Input: part model. Units: mm. Frame: model coordinates. Face numbers are marked on the shaded views. A direction names the side the tool comes from. Give positions to 0.01 mm unless a question says otherwise; leave off trailing zeros. Order: outer loops, then holes, each group sorted by start corner. A loop starts at its lowest first (then second) coordinate and runs counter-clockwise, first axis right, second up. Notation, with made-up numbers: (-18.75, -29.75) - (30.25, -29.75) arc R23 cw to (30.25, -19.75) - close; hole circle Ø1 at (23.5, 9.5). An arc over 180 degrees is marked (long way). Use a Markdown table: item, result.
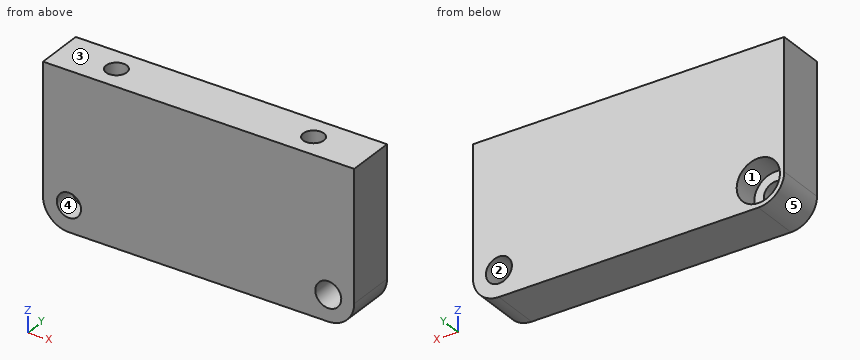
from build123d import *

# Parameters (mm, degrees)
SKETCH_1_W          = 180
SKETCH_1_H          = 28
EXTRUDE_1_DEPTH     = 90
SKETCH_2_R          = 6
CUT_EXTRUDE_1_DEPTH = 60
SKETCH_3_R          = 12.5
SKETCH_3_R_2        = 7.5
CUT_EXTRUDE_2_DEPTH = 30
FILLET_1_R          = 15
EXTRUDE_START       = -13
SKETCH_4_R          = 12.5
SKETCH_4_R_2        = 7
EXTRUDE_2_DEPTH     = 13


with BuildPart() as part:
    # 草图1 → 拉伸1 (new body)
    with BuildSketch(Plane.XY):
        with Locations((90, -14)):
            Rectangle(SKETCH_1_W, SKETCH_1_H)
    extrude(amount=EXTRUDE_1_DEPTH)

    # 草图2 → 切除-拉伸1 (cut)
    with BuildSketch(Plane.XY.offset(90)):
        with Locations((33, -14)):
            Circle(SKETCH_2_R)
        with Locations((147, -14)):
            Circle(SKETCH_2_R)
    extrude(amount=-CUT_EXTRUDE_1_DEPTH, mode=Mode.SUBTRACT)

    # 草图3 → 切除-拉伸2 (cut)
    with BuildSketch(Plane(origin=(0, 0, 0), x_dir=(1, 0, 0), z_dir=(0, 1, 0))):
        with Locations(Location((15, -15, 0), (0, 0, 270))):
            Circle(SKETCH_3_R)
        with Locations(Location((165, -15, 0), (0, 0, 270))):
            Circle(SKETCH_3_R_2)
    extrude(amount=-CUT_EXTRUDE_2_DEPTH, mode=Mode.SUBTRACT)

    # 圆角1
    fillet_1_edges = [part.edges().sort_by_distance(p)[0] for p in [
        (180, -14, 0),
        (0, -14, 0),
    ]]
    fillet(fillet_1_edges, radius=FILLET_1_R)

    # 草图4 → 拉伸2 (add)
    with BuildSketch(Plane.XZ.offset(28).offset(EXTRUDE_START)):
        with Locations(Location((15, 15, 0), (0, 0, 90))):
            Circle(SKETCH_4_R)
        with Locations(Location((15, 15, 0), (0, 0, 270))):
            Circle(SKETCH_4_R_2, mode=Mode.SUBTRACT)
    extrude(amount=EXTRUDE_2_DEPTH)


solid = part.part
1. Section query A-A (x = 13). Return loops of the section in (y, z).
Response:
| item | result |
|---|---|
| outline | (-28, 0.13) - (0, 0.13) - (0, 2.66) - (-15, 2.66) - (-15, 8.29) - (-28, 8.29) - close; (-28, 21.71) - (-15, 21.71) - (-15, 27.34) - (0, 27.34) - (0, 90) - (-28, 90) - close |
2. Mould query, pull axis X, two halves, no side actions, for the marked faces 3, 4 and 5. Classes: pulls with the +X half, pulls with the -X half, needs draft (parallel to the pull), parting line crosses it, or undercut.
Response:
| item | result |
|---|---|
| face 3 | needs draft |
| face 4 | undercut |
| face 5 | pulls with the -X half |
3. Section query B-B (z = 25). Return loops of the section in (x, y).
Response:
| item | result |
|---|---|
| outline | (0, -28) - (180, -28) - (180, 0) - (22.5, 0) - (22.5, -15) - (7.5, -15) - (7.5, 0) - (0, 0) - close |
4. Section query D-D (x = 147). Return loops of the section in (y, z), then the cut area to 3 significant figures.
Response:
| item | result |
|---|---|
| outline | (-28, 0) - (0, 0) - (0, 90) - (-8, 90) - (-8, 30) - (-20, 30) - (-20, 90) - (-28, 90) - close |
| area | 1,800 mm^2 |
5. Section query C-C (y = -2). Return loops of the section in (x, z), then the cut area to 3 significant figures.
Response:
| item | result |
|---|---|
| outline | (0, 15) arc R15 ccw to (15, 0) - (165, 0) arc R15 ccw to (180, 15) - (180, 90) - (0, 90) - close; hole circle Ø25 at (15, 15); hole circle Ø15 at (165, 15) |
| area | 15,400 mm^2 |
6. Pin query (flat end, axial travel): pin 1 (8.5 mm diameter, centred on x = 15, z = 15, fed in from -Y); pin 2 (7.5 mm diameter, centred on x = 9, z = 11, fed in from +Y). Return the tip coordinate at first contact, or that it passes through.
Response:
| item | result |
|---|---|
| pin 1 | passes through |
| pin 2 | stops at y = -15 |
7. Set-up query: the marked faces 1 and 2. Return all of +Z, -Z, +X, -X, +Y, -Y with unobstructed straight access to the full face (end or side cutting, diameter ignored); none if empty.
Response:
| item | result |
|---|---|
| face 1 | +Y |
| face 2 | +Y, -Y |
8. Material intervals for line 1 along X through (y, z) = (-11.75, 15); line 2 along X through (y, z) = (-17, 15.5); line 3 along Y through (x, z) = (147, 77), sorted ascending.
Response:
| item | result |
|---|---|
| line 1 | x = 0 to 2.5, 27.5 to 157.5, 172.5 to 180 |
| line 2 | x = 0 to 8.02, 21.98 to 157.52, 172.48 to 180 |
| line 3 | y = -28 to -20, -8 to 0 |
